```python
from build123d import *

# Parameters (mm, degrees)
BOSS_EXTRUDE1_DEPTH = 3


with BuildPart() as part:
    # Sketch1 → Boss-Extrude1 (new body)
    with BuildSketch(Plane(origin=(0, 0, 0), x_dir=(1, 0, 0), z_dir=(0, 1, 0))):
        Polygon((68.526631134, -52.5), (68.526631134, -60), (190, -60), (190, 60), (68.526631134, 60), (68.526631134, 52.5), (62.526631134, 52.5), (62.526631134, 40.526631134), (55, 33), (35, 33), (27.473368866, 40.526631134), (27.473368866, 52.5), (19.973368866, 52.5), (0, 32.526631134), (0, 23), (40, 23), (40, -23), (0, -23), (0, -32.526631134), (19.973368866, -52.5), (27.473368866, -52.5), (27.473368866, -40.526631134), (35, -33), (55, -33), (62.526631134, -40.526631134), (62.526631134, -52.5), align=None)
    extrude(amount=BOSS_EXTRUDE1_DEPTH)


solid = part.part
```
Work out the finished part from the listing and answer in its coordinate system (mm). A direction names the side the tool comes from. Give positions to 0.01 mm unless a question says otherwise; leave off trailing zeros. Loops run counter-clockwise (first coordinate to the right, second up) from the corner with the lowest first, then second, coordinate; pieces in that order, holes last. Notation, with made-up numbers: (-34, 81.25) -> (-14, 81.25) arc R28 cw to (-14, 114.25) -> close; hole circle Ø7 at (31.25, 78.25). An arc over 180 degrees is marked (long way). Put each result on its own line as item: value. Start each with the question number.
Item 1: The part is cut by section A-A (z = -46). Give the vertices of the cut face in (x, y).
Item 2: The part is cut by section B-B (y = 1). Give the vertices of the cut face in (x, z), then the cut area to 3 significant figures.
Item 3: Each of these flat-tipped pins is pushed along its axis until it touches: P1, Ø1.5, axis at x = 38.5, z = -35.5, coming from the -Y side; P2, Ø1.5, axis at x = 48, y = 2, coming from the -Z side; P3, Ø0.9, axis at x = 46.5, y = 1.5, coming from the +Z side; P4, Ø1.5, axis at x = 25.5, y = 1, coming from the +Z side. Where does it stop, or does it pass through?
Item 4: The mould has two halves that part along X. Classify faces 1 (the face through (115, 0, -1)), 2 (the face through (59, 1, -37)), 3 (the face through (9.847, 1.479, 42.374)): released by +X, released by -X, zero draft, split by the parting line, or undercut.
Item 5: Which of the six approach directions +Z, -Z, +X, -X, +Y, -Y give full straight-line access (tool end or side, diameter ignored) to faces 4 (the face through (59, 1, 37)), 5 (the face through (31, 1, -37)), 6 (the face through (10.126, 1.479, -42.653))?
Item 6: Find the intervals of material crossed by L1, parallel to X at y = 0.9, z = 49; L2, parallel to X at y = 0.9, z = -46.5; L3, parallel to Z at x = 48, y = 0.35, in increasing order. Write a range as [from, to].
Item 7: The part is cut by section C-C (z = 19). Give the vertices of the cut face in (x, y).
Answers below:
1. outline: (13.47, 0) -> (27.47, 0) -> (27.47, 3) -> (13.47, 3) -> close; (62.53, 0) -> (190, 0) -> (190, 3) -> (62.53, 3) -> close
2. outline: (0, -32.53) -> (19.97, -52.5) -> (27.47, -52.5) -> (27.47, -40.53) -> (35, -33) -> (55, -33) -> (62.53, -40.53) -> (62.53, -52.5) -> (68.53, -52.5) -> (68.53, -60) -> (190, -60) -> (190, 60) -> (68.53, 60) -> (68.53, 52.5) -> (62.53, 52.5) -> (62.53, 40.53) -> (55, 33) -> (35, 33) -> (27.47, 40.53) -> (27.47, 52.5) -> (19.97, 52.5) -> (0, 32.53) -> (0, 23) -> (40, 23) -> (40, -23) -> (0, -23) -> close
2. area: 18,300 mm2
3. P1: through
3. P2: z = -33
3. P3: z = 33
3. P4: z = 52.5
4. face 1: zero draft
4. face 2: undercut
4. face 3: released by -X
5. face 4: +Z, +Y, -Y
5. face 5: -Z, +Y, -Y
5. face 6: -Z, -X, +Y, -Y
6. L1: [16.47, 27.47], [62.53, 190]
6. L2: [13.97, 27.47], [62.53, 190]
6. L3: [-33, 33]
7. outline: (40, 0) -> (190, 0) -> (190, 3) -> (40, 3) -> close
